Here's how the part is built. I have some questions about the finished solid (model axes, mm). Face numbers are marked on the shaded views. Round coordinates to 2 decimals unless told otherwise and drop trailing zeros. Loops run counter-clockwise (first coordinate to the right, second up) from the corner with the lowest first, then second, coordinate; pieces in that order, holes last. Notation, with made-up numbers: (35, 0) - (48, 0) arc R5 ccw to (48, 8) - close; hole circle Ø9 at (12.25, 30.5). An arc over 180 degrees is marked (long way). Return JSON: item names as keys, results as strings. Group by question number.
```python
from build123d import *

# Parameters (mm, degrees)
F1_DEPTH = 25.4


with BuildPart() as f1:
    # F0 (on Front) → F1 (new body)
    with BuildSketch(Plane.XZ):
        with BuildLine():
            Line((-36.8707050923, 67.6275), (36.8707050923, 67.6275))
            ThreePointArc((36.8707050923, 67.6275), (26.5741043582, 72.2962283097), (15.705, 75.4074308358))
            Line((15.705, 75.4074308358), (15.705, 73.1806760713))
            ThreePointArc((15.705, 73.1806760713), (12.5580129473, 70.1790324087), (9.7084178523, 73.4643330011))
            Line((9.7084178523, 73.4643330011), (9.7084178523, 76.4112182409))
            ThreePointArc((9.7084178523, 76.4112182409), (-0.0017087982, 77.025499981), (-9.7118081837, 76.4107874063))
            Line((-9.7118081837, 76.4107874063), (-9.7118081837, 73.498063325))
            ThreePointArc((-9.7118081837, 73.498063325), (-9.699204988, 73.3395920741), (-9.695, 73.1806760713))
            ThreePointArc((-9.695, 73.1806760713), (-12.7, 70.1756760713), (-15.705, 73.1806760713))
            Line((-15.705, 73.1806760713), (-15.705, 75.4074308358))
            ThreePointArc((-15.705, 75.4074308358), (-26.5741043582, 72.2962283097), (-36.8707050923, 67.6275))
        make_face()
    extrude(amount=F1_DEPTH)


solid = f1.part
```
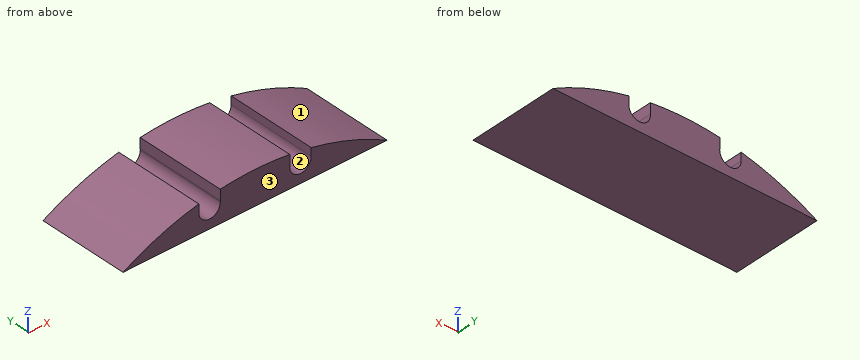
Q1. Will this pin go through, and if not, where does the flat tip stop? pin 1 Ø1.5 at (y, z) = (-16, 71.5) entering from -X.
Q2. Imagine slicing it at D-D, the plane z = 69. List the corners of the cut face in (x, y) for me, and give its area (3 significant figures).
Q3. Please list where these lines run through material, in increasing order: line 1 (X direction, y = -12.75, z = 70.5); line 2 (X direction, y = -17.5, z = 70.75); line 3 (Z direction, x = -1, y = -13.75).
Q4. If we mould it in two halves opening along X, with no side actions, what happens to the marked faces 1, 2 and 3? For each: +X half, -X half, draft (parallel to the pull), parting line (faces both ways), or undercut.
Q5. Imagine slicing it at B-B, the plane z = 72.5. List the corners of the cut face in (x, y) for me, and give its area (3 significant figures).
Q6. Imagine slicing it at A-A, the plane y = -10.5. List the corners of the cut face in (x, z) for me (1 decimal).
Q7. Imagine slicing it at C-C, the plane x = 7.5. List the corners of the cut face in (y, z) for me, and give its area (3 significant figures).
Output values:
{
 "1": {"pin 1": "stops at x = -30.45"},
 "2": {"outline": "(-34.23, -25.4) - (34.23, -25.4) - (34.23, 0) - (-34.23, 0) - close", "area": "1,740 mm^2"},
 "3": {"line 1": "x = -31.03 to -14.06, -11.34 to 11.34, 14.06 to 31.03", "line 2": "x = -30.45 to -14.47, -10.93 to 10.93, 14.47 to 30.45", "line 3": "z = 67.63 to 77.02"},
 "4": {"face 1": "+X half", "face 2": "undercut", "face 3": "draft"},
 "5": {"outline": "(-26.01, -25.4) - (-15.63, -25.4) - (-15.63, 0) - (-26.01, 0) - close; (-9.77, -25.4) - (9.77, -25.4) - (9.77, 0) - (-9.77, 0) - close; (15.63, -25.4) - (26.01, -25.4) - (26.01, 0) - (15.63, 0) - close", "area": "1,020 mm^2"},
 "6": {"outline": "(-36.9, 67.6) - (36.9, 67.6) arc R77 ccw to (15.7, 75.4) - (15.7, 73.2) arc R3 cw (long way) to (9.7, 73.5) - (9.7, 76.4) arc R77 ccw to (-9.7, 76.4) - (-9.7, 73.5) arc R3 cw (long way) to (-15.7, 73.2) - (-15.7, 75.4) arc R77 ccw to start"},
 "7": {"outline": "(-25.4, 67.63) - (0, 67.63) - (0, 76.66) - (-25.4, 76.66) - close", "area": "229 mm^2"}
}
